For this review, take the finished solid that the model builds, in its own axes (mm). A direction names the side the tool comes from. Round coordinates to 2 decimals unless told otherwise and drop trailing zeros. Order: outer loops, then holes, each group sorted by start corner. A loop starts at its lowest first (then second) coordinate and runs counter-clockwise, first axis right, second up. Notation, with made-up numbers: (55.25, 70.25) -> (88.25, 70.25) arc R28 ccw to (88.25, 91.25) -> close; hole circle Ø2 at (48.5, 82). An arc over 180 degrees is marked (long way). Answer in a Markdown table with one row per item.
```python
from build123d import *

# Parameters (mm, degrees)
SKETCH1_W           = 127
SKETCH1_H           = 127
BOSS_EXTRUDE1_DEPTH = 15.24
SKETCH2_W           = 127
SKETCH2_H           = 127
SKETCH2_W_2         = 100.33
SKETCH2_H_2         = 100.33
CUT_EXTRUDE1_DEPTH  = 6.35


with BuildPart() as part:
    # Sketch1 → Boss-Extrude1 (new body)
    with BuildSketch(Plane(origin=(0, 0, 0), x_dir=(1, 0, 0), z_dir=(0, 1, 0))):
        Rectangle(SKETCH1_W, SKETCH1_H)
    extrude(amount=BOSS_EXTRUDE1_DEPTH)

    # Sketch2 → Cut-Extrude1 (cut)
    with BuildSketch(Plane.XZ):
        Rectangle(SKETCH2_W, SKETCH2_H)
        Rectangle(SKETCH2_W_2, SKETCH2_H_2, mode=Mode.SUBTRACT)
    extrude(amount=-CUT_EXTRUDE1_DEPTH, mode=Mode.SUBTRACT)


solid = part.part
```
Q1. Clearance check with a flat-ended pin moving along its axis: pin 1 Ø7 at (x, y) = (-20, 2.5) entering from -Z (3 decimals). State where the tip first meets the part, or that it passes through.
Answer key:
| item | result |
|---|---|
| pin 1 | stops at z = -50.165 |
Q2. Tool access review of faces 1 (the face through (50.165, 3, -1)), 2 (the face through (-1, 15.24, -1)), 3 (the face through (-1, 3, 50.165)), 4 (the face through (-1, 3, -50.165)), 5 (the face through (-50.165, 3, -1)): name each direction out of +Z, -Z, +X, -X, +Y, -Y from which nothing blocks a thin tool from reaching the whole face with its end or side.
Answer key:
| item | result |
|---|---|
| face 1 | +Z, -Z, +X, -Y |
| face 2 | +Z, -Z, +X, -X, +Y |
| face 3 | +Z, +X, -X, -Y |
| face 4 | -Z, +X, -X, -Y |
| face 5 | +Z, -Z, -X, -Y |
Q3. Take a section at D-D, the plane x = -52.5. Write out the cut boundary in (y, z), then the cut area to 3 significant figures.
Answer key:
| item | result |
|---|---|
| outline | (6.35, -63.5) -> (15.24, -63.5) -> (15.24, 63.5) -> (6.35, 63.5) -> close |
| area | 1,130 mm^2 |
Q4. Take a section at B-B, the plane z = 26. Write out the cut boundary in (x, y) (3 decimals), then the cut area to 3 significant figures.
Answer key:
| item | result |
|---|---|
| outline | (-63.5, 6.35) -> (-50.165, 6.35) -> (-50.165, 0) -> (50.165, 0) -> (50.165, 6.35) -> (63.5, 6.35) -> (63.5, 15.24) -> (-63.5, 15.24) -> close |
| area | 1,770 mm^2 |
Q5. Take a section at C-C, the plane y = 3. Write out the cut boundary in (x, z) (3 decimals).
Answer key:
| item | result |
|---|---|
| outline | (-50.165, -50.165) -> (50.165, -50.165) -> (50.165, 50.165) -> (-50.165, 50.165) -> close |
Q6. To check wall thickness, follow probe 1 along X at (y, z) = (1.5, -0.5) (3 decimals); probe 2 along Y at (x, z) = (-23.5, -57.5). State the ranges of each line that lie inside material, in increasing order.
Answer key:
| item | result |
|---|---|
| probe 1 | x = -50.165 to 50.165 |
| probe 2 | y = 6.35 to 15.24 |
Q7. Take a section at A-A, the plane x = 39. Write out the cut boundary in (y, z) (3 decimals).
Answer key:
| item | result |
|---|---|
| outline | (0, -50.165) -> (6.35, -50.165) -> (6.35, -63.5) -> (15.24, -63.5) -> (15.24, 63.5) -> (6.35, 63.5) -> (6.35, 50.165) -> (0, 50.165) -> close |
